from build123d import *

# Parameters (mm, degrees)
PAD_DEPTH = 4


with BuildPart() as part:
    # Sketch → Pad (new body)
    with BuildSketch(Plane.XY):
        with BuildLine():
            ThreePointArc((-1.4, 2.428286), (0, -1), (1.4, 2.428286))
            Line((1.4, 2.428286), (4.883254, 2.985357))
            ThreePointArc((4.883254, 2.985357), (6.633254, -1.3), (8.383254, 2.985357))
            Line((8.383254, 2.985357), (9.946507, 4.39098))
            ThreePointArc((3.073564, -1.713522), (9.687991, -2.23927), (9.946507, 4.39098))
            ThreePointArc((-3.789459, 2.565248), (-2.169123, -2.479211), (3.073564, -1.713522))
            Line((-3.789459, 2.565248), (-1.4, 2.428286))
        make_face()
    extrude(amount=PAD_DEPTH)


solid = part.part
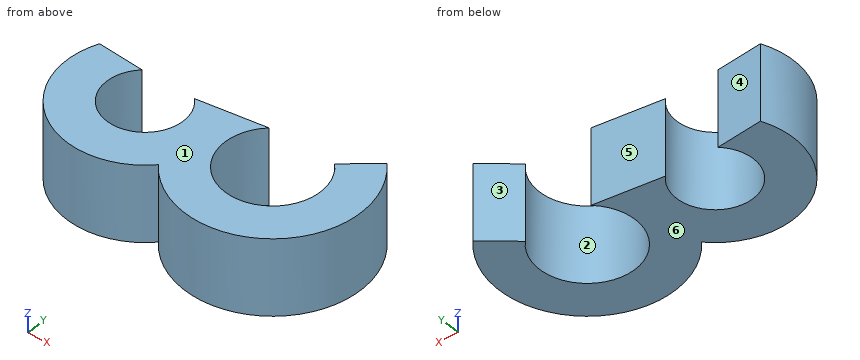
Model file for the job. Use its own axes, mm. Face numbers are marked on the shaded views. A direction names the side the tool comes from. Give positions to 0.01 mm unless a question says otherwise; leave off trailing zeros. Order: outer loops, then holes, each group sorted by start corner. A loop starts at its lowest first (then second) coordinate and runs counter-clockwise, first axis right, second up. Notation, with made-up numbers: M -24.5,82.25 L -12.5,82.25 A12 ccw -12.5,90.25 Z; hole C -34.75,-27.75 d1. An arc over 180 degrees is marked long. Put each result on its own line as item: value. Start each with the question number.
(1) Pin check, flat tips, straight feed: pin 1 Ø2 at (y, z) = (-1, 2.5) entering from -X; pin 2 Ø2.5 at (x, y) = (0, 1) entering from +Z. Stop position of each tip, or through.
(2) Pull direction X, two halves, no side cores. Call the marked faces 1, 2, 3 and 4: released by +X, released by -X, zero draft, split by the parting line, or undercut.
(3) Tool access for the marked faces 5 and 6: list every direction of +Z, -Z, +X, -X, +Y, -Y with a clear straight run to the whole face (end or side of a thin tool).
(4) Band-saw the part on B-B on y = -2.75. Give the cut face in (x, z), then the cut area to 3 significant figures.
(5) Band-saw the part on C-C on z = 1.05. Give the cut face in (x, y), then the cut area to 3 significant figures.
(6) Band-saw the part on A-A on y = 1. Give the cut face in (x, z), then the cut area to 3 significant figures.
(7) Band-saw the part on D-D on x = 7. Give the cut face in (y, z).
(8) Drill centre lines: L1, parallel to X at y = 1.2, z = 2.8; L2, parallel to X at y = 2, z = 1.9; L3, parallel to Y at x = 4.5, z = 0.85. Where is each one in solid material? Low to high. Write a range as [from, to].
Results below:
1. pin 1: stops at x = -3.98
1. pin 2: passes through
2. face 1: zero draft
2. face 2: undercut
2. face 3: released by -X
2. face 4: undercut
3. face 5: +Z, -Z, +Y
3. face 6: -Z, +X, -X, +Y, -Y
4. outline: M -1.66,0 L 1.66,0 L 1.66,4 L -1.66,4 Z; M 4.28,0 L 8.99,0 L 8.99,4 L 4.28,4 Z
4. area: 32.1 mm2
5. outline: M -3.79,2.57 A4.1 ccw 3.07,-1.71 A4.6 ccw long 9.95,4.39 L 8.38,2.99 A2.5 cw long 4.88,2.99 L 1.4,2.43 A2 cw long -1.4,2.43 Z
5. area: 52.7 mm2
6. outline: M -4.1,0 L -2,0 L -2,4 L -4.1,4 Z; M 2,0 L 4.14,0 L 4.14,4 L 2,4 Z; M 9.13,0 L 11.23,0 L 11.23,4 L 9.13,4 Z
6. area: 25.4 mm2
7. outline: M -3.39,0 L -1.27,0 L -1.27,4 L -3.39,4 Z
8. L1: x = [-4.1, -1.99], [1.99, 4.13], [9.13, 11.23]
8. L2: x = [-3.98, -1.73], [1.73, 4.26], [9, 11.16]
8. L3: y = [-2.88, -0.1], [2.5, 2.92]
